Verification items for the finished model (mm, model axes). A direction names the side the tool comes from. Coordinates: 2 decimals unless noted, no trailing zeros. Write each loop counter-clockwise with the first axis right and the second up, starting at its lowest first coordinate (ties: lowest second). Pieces come first, ordered by that corner, then holes. Notation, with made-up numbers: (-36, 36.5) - (-31, 36.5) arc R23 ccw to (-31, 63.5) - close; hole circle Ø8 at (78, 15). An arc over 180 degrees is marked (long way). Use one line per item in the form item = value. Start each with the question number.
(1) Tool access check on faces 1 (the cylindrical face through (1.802, 14.07, 5.723)), 2 (the cylindrical face through (-2.44, 9.86, -0.54)). Record the directions out of +Z, -Z, +X, -X, +Y, -Y that give a thin tool (end or side, any length) a straight path to the whole face; none if there is none.
(2) Sectioned sample at D-D (x = 3.5). Record the cut outline in (y, z).
(3) Sectioned sample at A-A (x = 0). Record the cut outline in (y, z).
(4) Mould release check, pull along Y, two halves, no side actions. Record for faces 3 (the flat face through (0, 20, 3)), 4 (the flat face through (2, 9, 6)), 5 (the cylindrical face through (-3.955, 4.437, -5.158)): released by +Y, released by -Y, zero draft, split by the parting line, or undercut.
(5) Material ranges on line 1 (Y direction, x = -5.5, z = -3.25); line 2 (X direction, y = 8.25, z = 0); line 3 (X direction, y = 12.75, z = 0), recorded low to high. Write a range as [from, to].
(6) Sectioned sample at C-C (y = 10.25). Record the cut outline in (x, z).
(7) Sectioned sample at B-B (z = 0). Record the cut outline in (x, y), and give its area (3 significant figures).
(8) Gauge pin test, flat ends, axial feed: pin 1 Ø6 at (x, y) = (-3, 11.5) entering from -Z; pin 2 Ø6 at (x, y) = (1, 12.5) entering from +Z; pin 3 Ø4 at (y, z) = (9.5, 4) entering from -X. Record the tip position at first contact, or that the pin passes through.
from build123d import *

# Parameters (mm, degrees)
SKETCH1_R           = 6.5
SKETCH1_R_2         = 2.5
BOSS_EXTRUDE1_DEPTH = 20
SKETCH2_R           = 6.793151268
SKETCH2_R_2         = 6
CUT_EXTRUDE1_DEPTH  = 10


with BuildPart() as part:
    # Sketch1 → Boss-Extrude1 (new body)
    with BuildSketch(Plane(origin=(0, 0, 0), x_dir=(1, 0, 0), z_dir=(0, 1, 0))):
        with Locations(Location((0, 0, 0), (0, 0, 270))):
            Circle(SKETCH1_R)
        with Locations(Location((0, 0, 0), (0, 0, 270))):
            Circle(SKETCH1_R_2, mode=Mode.SUBTRACT)
    extrude(amount=BOSS_EXTRUDE1_DEPTH)

    # Sketch2 → Cut-Extrude1 (cut)
    with BuildSketch(Plane(origin=(0, 19, 0), x_dir=(1, 0, 0), z_dir=(0, 1, 0))):
        Circle(SKETCH2_R)
        with Locations(Location((0, 0, 0), (0, 0, 270))):
            Circle(SKETCH2_R_2, mode=Mode.SUBTRACT)
    extrude(amount=-CUT_EXTRUDE1_DEPTH, mode=Mode.SUBTRACT)


solid = part.part
Answers below:
q1.face_1 = none
q1.face_2 = +Y, -Y
q2.outline = (0, -5.48) - (9, -5.48) - (9, -4.87) - (19, -4.87) - (19, -5.48) - (20, -5.48) - (20, 5.48) - (19, 5.48) - (19, 4.87) - (9, 4.87) - (9, 5.48) - (0, 5.48) - close
q3.outline = (0, -6.5) - (9, -6.5) - (9, -6) - (19, -6) - (19, -6.5) - (20, -6.5) - (20, -2.5) - (0, -2.5) - close; (0, 2.5) - (20, 2.5) - (20, 6.5) - (19, 6.5) - (19, 6) - (9, 6) - (9, 6.5) - (0, 6.5) - close
q4.face_3 = released by +Y
q4.face_4 = undercut
q4.face_5 = zero draft
q5.line_1 = [0, 9], [19, 20]
q5.line_2 = [-6.5, -2.5], [2.5, 6.5]
q5.line_3 = [-6, -2.5], [2.5, 6]
q6.outline = circle Ø12 at (0, 0); hole circle Ø5 at (0, 0)
q7.outline = (-6.5, 0) - (-2.5, 0) - (-2.5, 20) - (-6.5, 20) - (-6.5, 19) - (-6, 19) - (-6, 9) - (-6.5, 9) - close; (2.5, 0) - (6.5, 0) - (6.5, 9) - (6, 9) - (6, 19) - (6.5, 19) - (6.5, 20) - (2.5, 20) - close
q7.area = 150 mm2
q8.pin_1 = -6.36
q8.pin_2 = 6
q8.pin_3 = -6.16
